Source: CAD feature listing. Evaluate the final solid. Frame: model axes, mm. A direction names the side the tool comes from. Coordinates: 2 decimals unless noted, no trailing zeros. Loops run counter-clockwise (first coordinate to the right, second up) from the corner with the lowest first, then second, coordinate; pieces in that order, holes last. Notation, with made-up numbers: (-0.5, -26) - (30.5, -26) arc R34 cw to (30.5, 7) - close; hole circle Ø10 at (37, -14.75). An arc over 180 degrees is marked (long way). Use CSV: the item, a comma, the result in double quotes. Start each with the question number.
```python
from build123d import *

# Parameters (mm, degrees)
EXTRUDE_1_DEPTH          = 3
EXTRUDE_1_DEPTH_BACK     = 3
SKETCH_1_R               = 4
EXTRUDE_2_DEPTH          = 110.134
CUT_EXTRUDE_1_DEPTH      = 7
CUT_EXTRUDE_1_DEPTH_BACK = 7


with BuildPart() as part:
    # 草图1 → 凸台-拉伸1 (new, two sides: drawn at the far end of the back side and taken through both)
    with BuildSketch(Plane.XY.offset(-EXTRUDE_1_DEPTH_BACK)):
        with BuildLine():
            Line((-23.589809211, 8.747299509), (-5.474019211, -6.502700491))
            ThreePointArc((-5.474019211, -6.502700491), (-0.63908945, -8.475940342), (4.437059837, -7.25))
            Line((4.437059837, -7.25), (38.75, -7.25))
            Line((38.75, -7.25), (38.75, 11.05))
            Line((38.75, 11.05), (21.8949318, 11.05))
            Line((21.8949318, 11.05), (-15.462352545, 23.325225673))
            ThreePointArc((-15.462352545, 23.325225673), (-25.539933262, 19.389093721), (-23.589809211, 8.747299509))
        make_face()
        Circle(SKETCH_1_R, mode=Mode.SUBTRACT)
        with Locations((-18.11579, 15.25)):
            Circle(SKETCH_1_R, mode=Mode.SUBTRACT)
    extrude(amount=EXTRUDE_1_DEPTH + EXTRUDE_1_DEPTH_BACK)

    # 草图2 → 凸台-拉伸2 (add)
    with BuildSketch(Plane(origin=(38.75, 0, 0), x_dir=(0, 0, -1), z_dir=(1, 0, 0))):
        with BuildLine():
            Line((-7, 10.81), (-7, -6.19))
            ThreePointArc((-7, -6.19), (-5.535533906, -9.725533906), (-2, -11.19))
            Line((-2, -11.19), (2, -11.19))
            ThreePointArc((2, -11.19), (5.535533906, -9.725533906), (7, -6.19))
            Line((7, -6.19), (7, 10.81))
            ThreePointArc((7, 10.81), (5.535533906, 14.345533906), (2, 15.81))
            Line((2, 15.81), (-2, 15.81))
            ThreePointArc((-2, 15.81), (-5.535533906, 14.345533906), (-7, 10.81))
        make_face()
    extrude(amount=EXTRUDE_2_DEPTH)

    # 草图3 → 切除-拉伸1 (cut, two sides: drawn at the far end of the back side and taken through both)
    with BuildSketch(Plane.XY.offset(-CUT_EXTRUDE_1_DEPTH_BACK)):
        with BuildLine():
            Line((38.75, 15.81), (135.384, 15.81))
            ThreePointArc((135.384, 15.81), (148.881430926, 2.573359834), (135.910619432, -11.179724681))
            ThreePointArc((135.910619432, -11.179724681), (135.416543333, -11.158219373), (134.932713501, -11.055835964))
            ThreePointArc((134.932713501, -11.055835964), (126.070501893, -9.711605063), (117.183142857, -10.878052953))
            ThreePointArc((117.183142857, -10.878052953), (116.38, -10.987557918), (115.576857143, -10.878052953))
            ThreePointArc((115.576857143, -10.878052953), (106.886506673, -9.710238292), (98.205428571, -10.945092687))
            ThreePointArc((98.205428571, -10.945092687), (97.379999908, -11.060882627), (96.554571252, -10.945092637))
            ThreePointArc((96.554571252, -10.945092637), (87.873493235, -9.710238291), (79.183142857, -10.878052953))
            ThreePointArc((79.183142857, -10.878052953), (78.38, -10.987557918), (77.576857143, -10.878052953))
            ThreePointArc((77.576857143, -10.878052953), (68.676784071, -9.711734935), (59.802929496, -11.063142857))
            ThreePointArc((59.802929496, -11.063142857), (59.375984144, -11.158116286), (58.939766636, -11.19))
            Line((58.939766636, -11.19), (38.75, -11.19))
            Line((38.75, -11.19), (38.75, -16.19))
            Line((38.75, -16.19), (153.884, -16.19))
            Line((153.884, -16.19), (153.884, 20.81))
            Line((153.884, 20.81), (38.75, 20.81))
            Line((38.75, 20.81), (38.75, 15.81))
        make_face()
    extrude(amount=CUT_EXTRUDE_1_DEPTH + CUT_EXTRUDE_1_DEPTH_BACK, mode=Mode.SUBTRACT)


solid = part.part
```
(1) Draft query along X for faces 5 (the flat face through (-14.66, 1.23, -0.04)), 6 (the cylindrical face through (-14.3, 16.45, -0.04)), 7 (the flat face through (93, 2, -7)). Return one class per face: released by +X, released by -X, zero draft, split by the parting line, or undercut.
(2) Section C-C on x = 0. Output: boundary loops of the cut face in (y, z), plus the area to 3 significant figures.
(3) Ray query, line 1 (Z direction, x = 6, y = 3.5); line 2 (Y direction, x = 0, z = -0.25); line 3 (X direction, y = 2, z = 5.25). Return the intervals inside material, ascending. Write a range as [from, to].
(4) Section B-B on y = 0. Output: boundary loops of the cut face in (x, z).
(5) Pin query (flat end, axial travel): pin 1 Ø8 at (x, z) = (129, 3) entering from +Y; pin 2 Ø3 at (x, z) = (21, -1) entering from -Y; pin 3 Ø1.8 at (x, z) = (27.5, 0.5) entering from +Y. Return the tip coordinate at first contact, or that it passes through.
(6) Reachability of faces 1 (the flat face through (21, -7.25, 0)), 2 (the flat face through (3.48, 17.1, -0.04)), 3 (the flat face through (86, 15.81, 0)), 4 (the flat face through (6, 4, 3)) from +Z, -Z, +X, -X, +Y, -Y: full face, straight path, thin tool, end or side. Return the list, or none.
(7) Section A-A on z = 0. Output: boundary loops of the cut face in (x, y), plus the area to 3 significant figures.
Solution:
1,face 5,"released by -X"
1,face 6,"undercut"
1,face 7,"zero draft"
2,outline,"(-8.5, -3) - (-4, -3) - (-4, 3) - (-8.5, 3) - close; (4, -3) - (18.24, -3) - (18.24, 3) - (4, 3) - close"
2,area,"112 mm²"
3,line 1,"z = [-3, 3]"
3,line 2,"y = [-8.5, -4], [4, 18.24]"
3,line 3,"x = [38.75, 148.88]"
4,outline,"(-13.2, -3) - (-4, -3) - (-4, 3) - (-13.2, 3) - close; (4, -3) - (38.75, -3) - (38.75, -7) - (148.68, -7) - (148.68, 7) - (38.75, 7) - (38.75, 3) - (4, 3) - close"
5,pin 1,"stops at y = 15.81"
5,pin 2,"stops at y = -7.25"
5,pin 3,"stops at y = 11.05"
6,face 1,"+Z, -Z, -Y"
6,face 2,"+Z, -Z, +Y"
6,face 3,"+Z, -Z, +X, +Y"
6,face 4,"+Z, -X, +Y, -Y"
7,outline,"(-23.59, 8.75) - (-5.47, -6.5) arc R8.5 ccw to (4.44, -7.25) - (38.75, -7.25) - (38.75, -11.19) - (58.94, -11.19) arc R3 ccw to (59.8, -11.06) arc R32 cw to (77.58, -10.88) arc R3 ccw to (79.18, -10.88) arc R32 cw to (96.55, -10.95) arc R3 ccw to (98.21, -10.95) arc R32 cw to (115.58, -10.88) arc R3 ccw to (117.18, -10.88) arc R32 cw to (134.93, -11.06) arc R3 ccw to (135.91, -11.18) arc R13.5 ccw to (135.38, 15.81) - (38.75, 15.81) - (38.75, 11.05) - (21.89, 11.05) - (-15.46, 23.33) arc R8.5 ccw to start; hole circle Ø8 at (-18.12, 15.25); hole circle Ø8 at (0, 0)"
7,area,"4,070 mm²"
